from build123d import *

# Parameters (mm, degrees)
F0_W     = 1530
F0_H     = 2030
F1_DEPTH = 254
F2_R     = 50.8
F3_R     = 12.7
F4_W     = 1682.4
F4_H     = 2182.4
F5_DEPTH = 38.1
F6_W     = 152.4
F6_H     = 152.4
F7_DEPTH = 203.2
F7_TAPER = 5


with BuildPart() as f1:
    # F0 (on Top) → F1 (new body)
    with BuildSketch(Plane.XY):
        Rectangle(F0_W, F0_H)
    extrude(amount=F1_DEPTH)

    # F2
    f2_edges = [f1.edges().sort_by_distance(p)[0] for p in [
        (-765, -1015, 127),
        (765, -1015, 127),
        (765, 1015, 127),
        (-765, 1015, 127),
    ]]
    fillet(f2_edges, radius=F2_R)

    # F3
    f3_edges = [f1.edges().sort_by_distance(p)[0] for p in [
        (0, -1015, 254),
        (-750.121024, -1000.121024, 254),
        (750.121024, -1000.121024, 254),
        (-765, 0, 254),
        (765, 0, 254),
        (-750.121024, 1000.121024, 254),
        (750.121024, 1000.121024, 254),
        (0, 1015, 254),
        (0, -1015, 0),
        (-750.121024, -1000.121024, 0),
        (750.121024, -1000.121024, 0),
        (-765, 0, 0),
        (765, 0, 0),
        (-750.121024, 1000.121024, 0),
        (750.121024, 1000.121024, 0),
        (0, 1015, 0),
    ]]
    fillet(f3_edges, radius=F3_R)

    # F4 (on face) → F5 (join)
    with BuildSketch(Plane(origin=(0, 0, 0), x_dir=(1, 0, 0), z_dir=(0, 0, -1))):
        Rectangle(F4_W, F4_H)
    extrude(amount=F5_DEPTH)

    # F6 (on face) → F7 (join)
    with BuildSketch(Plane(origin=(0, 0, -38.1), x_dir=(1, 0, 0), z_dir=(0, 0, -1))):
        with Locations((-765, 1015)):
            Rectangle(F6_W, F6_H)
        with Locations((765, 1015)):
            Rectangle(F6_W, F6_H)
        with Locations((765, -1015)):
            Rectangle(F6_W, F6_H)
        with Locations((-765, -1015)):
            Rectangle(F6_W, F6_H)
    extrude(amount=F7_DEPTH, taper=F7_TAPER)


solid = f1.part
The listing builds one solid part. Answer for the finished solid, in the listing's coordinates (mm). A direction names the side the tool comes from. Coordinates: 2 decimals unless noted, no trailing zeros. Loops run counter-clockwise (first coordinate to the right, second up) from the corner with the lowest first, then second, coordinate; pieces in that order, holes last.
1) Flat-ended cylindrical pins translate along their axes: pin 1 Ø3 at (y, z) = (292, 187) entering from -X; pin 2 Ø1.5 at (x, z) = (605.5, 187) entering from -Y; pin 3 Ø8 at (y, z) = (448.5, 117.5) entering from +X. Find the tip coordinate at first contact, or state that the pin passes through.
2) Find section D-D on z = -83.5. Give the number of separate pieces and of enclosed holes in the cut face, then the cut area to 3 significant figures.
3) Find the intervals of material crossed by L1, parallel to Z at x = 577.5, y = 182.5; L2, parallel to Y at x = -682, z = 145.5; L3, parallel to X at y = 172.5, z = 85.5, in increasing order.
4) A tool of negligible diameter and unlimited length cuts with its end or side. For faces 1 (the face through (-765, -13, 125)), 2 (the face through (750.514, 999.724, 128.6)), 3 (the face through (765, -13, 125)), 4 (the face through (749.724, -1000.514, 128.6)), 5 (the face through (-12, -15, -38.1)), from which of +Z, -Z, +X, -X, +Y, -Y can it reach the whole face along a straight path? Write none if from no direction.
5) Find section B-B on y = 267. Write down the section's boundary in (x, z), then the cut area to 3 significant figures.
6) Find section A-A on z = 92. Write down the section's boundary in (x, y), then the cut area to 3 significant figures.
7) Find section C-C on x = 272. Write down the section's boundary in (y, z).
Values:
1. pin 1: stops at x = -765
1. pin 2: stops at y = -1015
1. pin 3: stops at x = 765
2. separate pieces: 4
2. enclosed holes: 0
2. area: 83,500 mm2
3. L1: z = -38.1 to 254
3. L2: y = -1015 to 1015
3. L3: x = -765 to 765
4. face 1: +Z, -X, +Y, -Y
4. face 2: +Z, +X, +Y
4. face 3: +Z, +X, +Y, -Y
4. face 4: +Z, +X, -Y
4. face 5: -Z
5. outline: (-841.2, -38.1) - (841.2, -38.1) - (841.2, 0) - (752.3, 0) arc R12.7 ccw to (765, 12.7) - (765, 241.3) arc R12.7 ccw to (752.3, 254) - (-752.3, 254) arc R12.7 ccw to (-765, 241.3) - (-765, 12.7) arc R12.7 ccw to (-752.3, 0) - (-841.2, 0) - close
5. area: 453,000 mm2
6. outline: (-765, -964.2) arc R50.8 ccw to (-714.2, -1015) - (714.2, -1015) arc R50.8 ccw to (765, -964.2) - (765, 964.2) arc R50.8 ccw to (714.2, 1015) - (-714.2, 1015) arc R50.8 ccw to (-765, 964.2) - close
6. area: 3,100,000 mm2
7. outline: (-1091.2, -38.1) - (1091.2, -38.1) - (1091.2, 0) - (1002.3, 0) arc R12.7 ccw to (1015, 12.7) - (1015, 241.3) arc R12.7 ccw to (1002.3, 254) - (-1002.3, 254) arc R12.7 ccw to (-1015, 241.3) - (-1015, 12.7) arc R12.7 ccw to (-1002.3, 0) - (-1091.2, 0) - close
